Build history of the part. All positions in model axes, mm. Face numbers are marked on the shaded views. Give positions to 0.01 mm unless a question says otherwise; leave off trailing zeros. Loops run counter-clockwise (first coordinate to the right, second up) from the corner with the lowest first, then second, coordinate; pieces in that order, holes last. Notation, with made-up numbers: (60, 16.25) -> (115, 16.25) arc R22 cw to (115, 42.25) -> close; hole circle Ø8 at (-6.75, 47). An arc over 180 degrees is marked (long way). Answer as a JSON object with one key per item and string values. Group by question number.
Q1. Drop flat-ended pins along their axis: pin 1 (4 mm diameter, centred on x = 18, y = -6, fed in from -Z); pin 2 (3 mm diameter, centred on x = -14.5, y = -10, fed in from +Z); pin 3 (1.5 mm diameter, centred on y = -12.5, z = 3, fed in from -X). Give the stop position or say it passes through.
Q2. Band-saw the part on A-A, the plane x = 0. Write the cut outline in (y, z) (3 decimals).
Q3. Band-saw the part on D-D, the plane y = -13. Write the cut outline in (x, z) (3 decimals).
Q4. Two-plate mould, pull along X, no slides. Class the marked faces 1, 2, 3 and 4: pulls with the +X half, pulls with the -X half, needs draft (parallel to the pull), parting line crosses it, or undercut.
Q5. Band-saw the part on B-B, the plane y = -7.62. Write the cut outline in (x, z) (3 decimals).
Q6. Band-saw the part on C-C, the plane z = 0. Write the cut outline in (x, y).
Q7. Wall check: probe 1 along Y at (x, z) = (0, -18) (3 decimals); probe 2 along Z at (x, y) = (-9, -8.75); probe 3 along X at (y, z) = (-23.75, 11.5). Give the ranges that are in metal, low to high. Write a range as from..to.
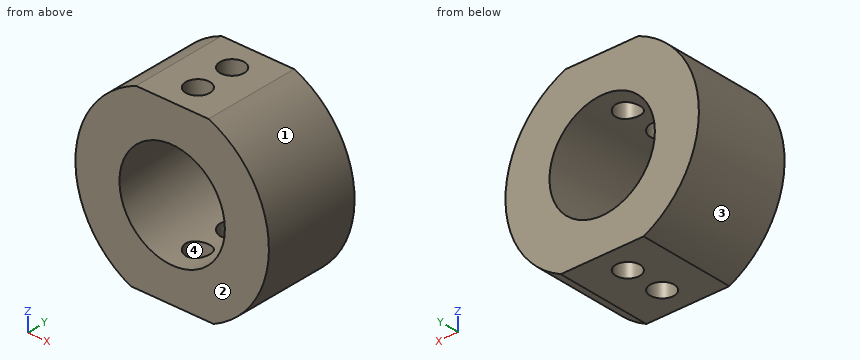
from build123d import *

# Parameters (mm, degrees)
F0_R     = 1.5875
F1_DEPTH = 25.4
F2_R     = 3.175
F2_R_2   = 3.161961
F3_DEPTH = 46.496531
F4_R     = 13.843
F5_DEPTH = 25.401


with BuildPart() as f1:
    # F0 (on Front) → F1 (new body)
    with BuildSketch(Plane.XZ):
        with BuildLine():
            Line((9.525, 23.54643), (-9.525, 23.54643))
            ThreePointArc((-9.525, 23.54643), (-25.38913, 0.743025), (-10.885714, -22.949101))
            Line((-10.885714, -22.949101), (10.885714, -22.949101))
            ThreePointArc((10.885714, -22.949101), (25.38913, 0.743025), (9.525, 23.54643))
        make_face()
        Circle(F0_R, mode=Mode.SUBTRACT)
    extrude(amount=F1_DEPTH)

    # F2 (on face) → F3 (cut, through all)
    with BuildSketch(Plane.XY.offset(23.54643)):
        with Locations((0, -7.62)):
            Circle(F2_R)
        with Locations((0, -17.78)):
            Circle(F2_R_2)
    extrude(amount=-F3_DEPTH, mode=Mode.SUBTRACT)

    # F4 (on face) → F5 (cut, through all)
    with BuildSketch(Plane.XZ.offset(25.4)):
        Circle(F4_R)
    extrude(amount=-F5_DEPTH, mode=Mode.SUBTRACT)


solid = f1.part
Worked answers:
{
 "1": {"pin 1": "z = -19.73", "pin 2": "z = 21.82", "pin 3": "x = -25.3"},
 "2": {"outline": "(-25.4, -22.949) -> (-20.942, -22.949) -> (-20.942, -13.843) -> (-25.4, -13.843) -> close; (-25.4, 13.843) -> (-20.942, 13.843) -> (-20.942, 23.546) -> (-25.4, 23.546) -> close; (-14.618, -22.949) -> (-10.795, -22.949) -> (-10.795, -13.843) -> (-14.618, -13.843) -> close; (-14.618, 13.843) -> (-10.795, 13.843) -> (-10.795, 23.546) -> (-14.618, 23.546) -> close; (-4.445, -22.949) -> (0, -22.949) -> (0, -13.843) -> (-4.445, -13.843) -> close; (-4.445, 13.843) -> (0, 13.843) -> (0, 23.546) -> (-4.445, 23.546) -> close"},
 "3": {"outline": "(-10.886, -22.949) -> (10.886, -22.949) arc R25.4 ccw to (9.525, 23.546) -> (-9.525, 23.546) arc R25.4 ccw to start; hole circle Ø27.686 at (0, 0)"},
 "4": {"face 1": "pulls with the +X half", "face 2": "needs draft", "face 3": "pulls with the -X half", "face 4": "undercut"},
 "5": {"outline": "(-10.886, -22.949) -> (-3.175, -22.949) -> (-3.175, -13.474) arc R13.843 cw to (-3.175, 13.474) -> (-3.175, 23.546) -> (-9.525, 23.546) arc R25.4 ccw to start; (3.175, -22.949) -> (10.886, -22.949) arc R25.4 ccw to (9.525, 23.546) -> (3.175, 23.546) -> (3.175, 13.474) arc R13.843 cw to (3.175, -13.474) -> close"},
 "6": {"outline": "(-25.4, -25.4) -> (-13.84, -25.4) -> (-13.84, 0) -> (-25.4, 0) -> close; (13.84, -25.4) -> (25.4, -25.4) -> (25.4, 0) -> (13.84, 0) -> close"},
 "7": {"probe 1": "-25.4..-20.942, -14.618..-10.795, -4.445..0", "probe 2": "-22.95..-10.52, 10.52..23.55", "probe 3": "-22.65..-7.71, 7.71..22.65"}
}
